Can you work these out from the model? Positions are in its coordinate system, mm. A direction names the side the tool comes from. Give positions to 0.01 mm unless a question says otherwise; leave off trailing zeros. Loops run counter-clockwise (first coordinate to the right, second up) from the corner with the lowest first, then second, coordinate; pieces in that order, holes last. Notation, with made-up numbers: M 60.5,61.25 L 114.5,61.25 A32 ccw 114.5,88.25 Z; hole C 50.25,-36 d11. An arc over 180 degrees is marked long. Put each result on its own line as item: value. Start each with the question number.
1) If we mould it in two halves opening along X, with no side actions, what happens to faces 4 (the cylindrical face through (0, -2, 2)), 5 (the flat face through (1, -1, 5)), 6 (the cylindrical face through (0, -1, 2))? For each: +X half, -X half, draft (parallel to the pull), parting line (faces both ways), or undercut.
2) Imagine slicing it at A-A (z = -1.75). Write out the boundary of the cut face in (x, y).
3) For P1, Ø2, axis at y = -1, z = 0.5, coming from the -X side, with a flat end and sliding along its axis, tell me the tip position at first contact or that it passes through.
4) For faces 1 (the flat face through (0.51, -0.86, -2.26)), 2 (the cylindrical face through (3, 0, -1)), 3 (the flat face through (-1, -2, 0)), which set-ups out of +Z, -Z, +X, -X, +Y, -Y let a thin tool reach every point of the face, with its end or its side?
5) Imagine slicing it at B-B (z = -0.5). Write out the boundary of the cut face in (x, y).
6) Imagine slicing it at C-C (z = 0.5). Write out the boundary of the cut face in (x, y), then the cut area to 3 significant figures.
7) Please list where these lines run through material, in increasing order: line 1 along Y through (x, z) = (0, 1); line 2 along Z through (x, y) = (1.15, -2); line 3 along X through (y, z) = (0.15, -2). Write a range as from..to.
from build123d import *

# Parameters (mm, degrees)
SKETCH1_R           = 2
BOSS_EXTRUDE1_DEPTH = 5
SKETCH2_R           = 3
BOSS_EXTRUDE2_DEPTH = 3
CHAMFER1_SIZE       = 0.5
CUT_EXTRUDE3_DEPTH  = 1.5
SKETCH6_R           = 1
CUT_EXTRUDE4_DEPTH  = 8.762087348


with BuildPart() as part:
    # Sketch1 → Boss-Extrude1 (new body)
    with BuildSketch(Plane.XY):
        Circle(SKETCH1_R)
    extrude(amount=BOSS_EXTRUDE1_DEPTH)

    # Sketch2 → Boss-Extrude2 (add)
    with BuildSketch(Plane(origin=(0, 0, 0), x_dir=(-1, 0, 0), z_dir=(0, 0, -1))):
        Circle(SKETCH2_R)
    extrude(amount=BOSS_EXTRUDE2_DEPTH)

    # Chamfer1
    chamfer1_edges = [part.edges().sort_by_distance(p)[0] for p in [
        (3, 0, -3),
    ]]
    chamfer(chamfer1_edges, length=CHAMFER1_SIZE)

    # Sketch5 → Cut-Extrude3 (cut)
    with BuildSketch(Plane(origin=(0, 0, -3), x_dir=(-1, 0, 0), z_dir=(0, 0, -1))):
        Polygon((0, -1.154700538), (1, -0.577350269), (1, 0.577350269), (0, 1.154700538), (-1, 0.577350269), (-1, -0.577350269), align=None)
    extrude(amount=-CUT_EXTRUDE3_DEPTH, mode=Mode.SUBTRACT)

    # Sketch6 → Cut-Extrude4 (cut, through all)
    with BuildSketch(Plane(origin=(0, 0, -1.5), x_dir=(-1, 0, 0), z_dir=(0, 0, -1))):
        Circle(SKETCH6_R)
    extrude(amount=-CUT_EXTRUDE4_DEPTH, mode=Mode.SUBTRACT)


solid = part.part
Recorded:
1. face 4: parting line
1. face 5: draft
1. face 6: undercut
2. outline: C 0,0 d6; hole M -1,-0.58 L 0,-1.15 L 1,-0.58 L 1,0.58 L 0,1.15 L -1,0.58 Z
3. P1: x = -3
4. face 1: -Z
4. face 2: +Z, -Z
4. face 3: +Z
5. outline: C 0,0 d6; hole C 0,0 d2
6. outline: C 0,0 d4; hole C 0,0 d2
6. area: 9.42 mm²
7. line 1: -2..-1, 1..2
7. line 2: -3..0
7. line 3: -3..-1, 1..3
